For this review, take the finished solid that the model builds, in its own axes (mm). Face numbers are marked on the shaded views. A direction names the side the tool comes from. Round coordinates to 2 decimals unless told otherwise and drop trailing zeros. Order: outer loops, then holes, each group sorted by start corner. A loop starts at its lowest first (then second) coordinate and runs counter-clockwise, first axis right, second up. Notation, with made-up numbers: (-20.5, 8) -> (25.5, 8) arc R9 cw to (25.5, 19) -> close; hole circle Ø3 at (2.25, 40.5). An arc over 180 degrees is marked (long way). Answer in a Markdown table with one row per item.
Autodesk Inventor part; units mm, degrees
ref_plane "YZ Plane" through (0, 0, 0) normal (1, 0, 0) x (0, 1, 0)
ref_plane "XZ Plane" through (0, 0, 0) normal (0, 1, 0) x (-1, 0, 0)
ref_plane "XY Plane" through (0, 0, 0) normal (0, 0, 1) x (1, 0, 0)
sketch "Sketch1" plane through (0, 0, 0) normal (0, 0, 1) x (1, 0, 0)
  line L0 (0, 4.4456) -> (0, -4.4456)
  line L1 (-3.85, 0) -> (3.85, 0)
  circle A0 centre (0, 0) radius 1.25
  line L2 (0, 3.1754) -> (2.75, 1.5877)
  line L3 (2.75, 1.5877) -> (2.75, -1.5877)
  line L4 (2.75, -1.5877) -> (0, -3.1754)
  line L5 (0, -3.1754) -> (-2.75, -1.5877)
  line L6 (-2.75, -1.5877) -> (-2.75, 1.5877)
  line L7 (-2.75, 1.5877) -> (0, 3.1754)
  dimension "d0" = 2.5
  dimension "d1" = 5.5
extrude "Extrusion1" add sketch "Sketch1" along normal mid plane 12
sketch "Sketch2" plane through (0, 0, -6) normal (0, 0, -1) x (-1, 0, 0)
  circle A0 centre (0, 0) radius 1.25
  dimension "d4" = 2.5
extrude "Extrusion2" cut sketch "Sketch2" against normal blind 4
sketch "Sketch3" plane through (2.75, -1.5877, 6) normal (1, 0, 0) x (0, 0, -1)
  line L0 (0, 3.1754) -> (0, 0)
  line L1 (12, 0) -> (0, 0)
  line L2 (12, 0) -> (12, 3.1754)
  line L3 (12, 3.1754) -> (0, 3.1754)
  line L4 (6, 0) -> (6, 3.1754)
  point P0 (6, 1.5877)
sketch "Sketch4" plane through (0, 0, 6) normal (0, 0, 1) x (1, 0, 0)
  line L0 (0, 3.1754) -> (2.75, 1.5877)
  line L1 (-2.75, 1.5877) -> (0, 3.1754)
  line L2 (-2.75, -1.5877) -> (-2.75, 1.5877)
  line L3 (0, -3.1754) -> (-2.75, -1.5877)
  line L4 (2.75, -1.5877) -> (0, -3.1754)
  line L5 (2.75, 1.5877) -> (2.75, -1.5877)
  circle A0 centre (0, 0) radius 1.25
  dimension "d7" = 2.5
extrude "Extrusion3" cut sketch "Sketch4" against normal blind 5
thread "Thread1"
thread "Thread2"
properties part number "Motherboard Standoff 11mm M3x0.5"
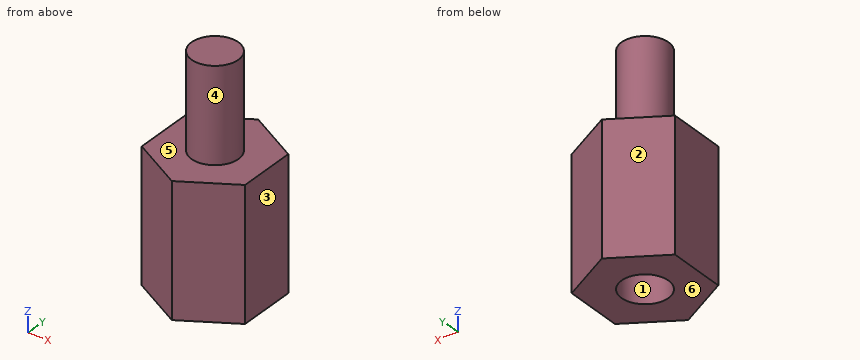
Q1. Tool access review of the marked faces 5 and 6: name each direction out of +Z, -Z, +X, -X, +Y, -Y from which nothing blocks a thin tool from reaching the whole face with its end or side.
Answer key:
| item | result |
|---|---|
| face 5 | +Z |
| face 6 | -Z, +X, -X, +Y, -Y |
Q2. Take a section at A-A, the plane z = -4.5. Write out the cut boundary in (x, y), then the cut area to 3 significant figures.
Answer key:
| item | result |
|---|---|
| outline | (-2.75, -1.59) -> (0, -3.18) -> (2.75, -1.59) -> (2.75, 1.59) -> (0, 3.18) -> (-2.75, 1.59) -> close; hole circle Ø2.5 at (0, 0) |
| area | 21.3 mm^2 |
Q3. Clearance check with flat-ended pins moving along their axes: pin 1 Ø1 at (x, y) = (1.5, 2.5) entering from +Z; pin 2 Ø1.5 at (y, z) = (-2.5, -4.5) entering from +X; pin 3 Ø1.5 at (x, z) = (0.5, -2.5) entering from +Y. State where each tip first meets the part, or that it passes through.
Answer key:
| item | result |
|---|---|
| pin 1 | stops at z = 1 |
| pin 2 | stops at x = 2.47 |
| pin 3 | stops at y = 3.18 |
Q4. To check wall thickness, follow probe 1 along Z at (x, y) = (-0.7, 1); probe 2 along Z at (x, y) = (0.75, 2.5); probe 3 along X at (y, z) = (-0.25, -4.5). State the ranges of each line that lie inside material, in increasing order.
Answer key:
| item | result |
|---|---|
| probe 1 | z = -2 to 6 |
| probe 2 | z = -6 to 1 |
| probe 3 | x = -2.75 to -1.22, 1.22 to 2.75 |
Q5. The part is to be moulded in two halves that separate along X. For the marked faces 1, 2, 3 and 4, say which applies: +X half, -X half, draft (parallel to the pull), parting line (faces both ways), or undercut.
Answer key:
| item | result |
|---|---|
| face 1 | undercut |
| face 2 | -X half |
| face 3 | +X half |
| face 4 | parting line |
Q6. Take a section at B-B, the plane y = 0. Write out the cut boundary in (x, z), then the cut area to 3 significant figures.
Answer key:
| item | result |
|---|---|
| outline | (-2.75, -6) -> (-1.25, -6) -> (-1.25, -2) -> (1.25, -2) -> (1.25, -6) -> (2.75, -6) -> (2.75, 1) -> (1.25, 1) -> (1.25, 6) -> (-1.25, 6) -> (-1.25, 1) -> (-2.75, 1) -> close |
| area | 41.0 mm^2 |
Q7. Take a section at D-D, the plane x = 0.6. Write out the cut boundary in (y, z).
Answer key:
| item | result |
|---|---|
| outline | (-2.83, -6) -> (-1.1, -6) -> (-1.1, -2) -> (1.1, -2) -> (1.1, -6) -> (2.83, -6) -> (2.83, 1) -> (1.1, 1) -> (1.1, 6) -> (-1.1, 6) -> (-1.1, 1) -> (-2.83, 1) -> close |
Q8. Take a section at C-C, the plane z = -0.5. Write out the cut boundary in (x, y).
Answer key:
| item | result |
|---|---|
| outline | (-2.75, -1.59) -> (0, -3.18) -> (2.75, -1.59) -> (2.75, 1.59) -> (0, 3.18) -> (-2.75, 1.59) -> close |
